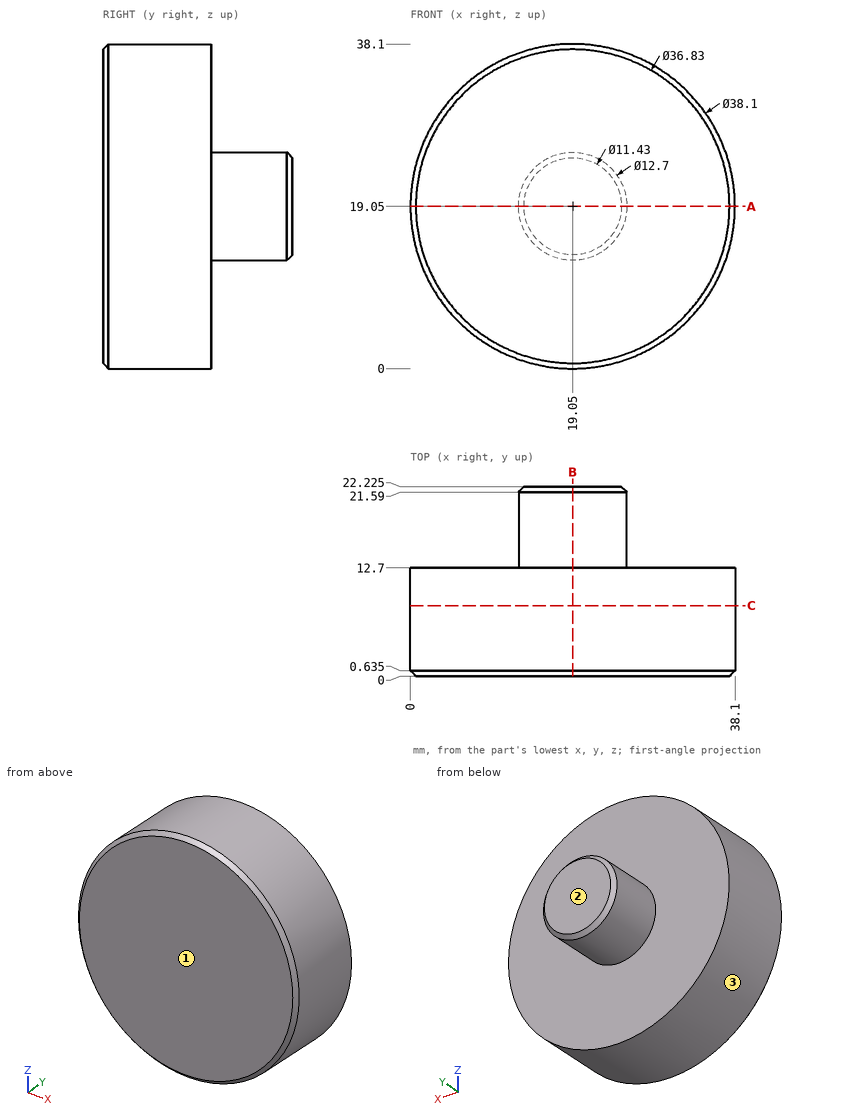
Check sheet for the drawn part. Datum: minimum x, y, z corner. Units: mm. Coordinates: 2 decimals unless noted, no trailing zeros. Order: outer loops, then holes, each group sorted by start corner. A loop starts at its lowest first (then second) coordinate and runs counter-clockwise, first axis right, second up. Notation, with made-up numbers: M 32,13.5 L 55,13.5 A30 ccw 55,41.5 Z; hole C 1,75.25 d4. An arc over 180 degrees is marked long. One line per question, with ' | ' between items. Start each with the question number.
Item 1: Gauge pin test, flat ends, axial feed: pin 1 (5 mm diameter, centred on y = 3, z = 25.5, fed in from -X); pin 2 (8 mm diameter, centred on y = 16.5, z = 16, fed in from +X); pin 3 (3 mm diameter, centred on x = 31, z = 24, fed in from +Y). Record the tip position at first contact, or that the pin passes through.
Item 2: Cross-section at B-B on x = 19.05. Enter the section's corners in (y, z) (3 decimals), then the cut area to 3 significant figures.
Item 3: Cross-section at C-C on y = 8.25. Enter the section's corners in (x, z), then the cut area to 3 significant figures.
Item 4: Cross-section at A-A on z = 19.05. Enter the section's corners in (x, y) (3 decimals), then the cut area to 3 significant figures.
Item 5: Material ranges on L1, parallel to Y at x = 21, z = 29; L2, parallel to Y at x = 9, z = 3.5; L3, parallel to Z at x = 33.5, y = 4.5, recorded low to high. Write a range as [from, to].
Item 6: Draft check along Y on the marked faces 1, 2 and 3. Enter one of: pulls with the +Y half, pulls with the -Y half, needs draft (parallel to the pull), parting line crosses it, or undercut.
Findings:
1) pin 1: stops at x = 0.41 | pin 2: stops at x = 38.01 | pin 3: stops at y = 12.7
2) outline: M 0,0.635 L 0.635,0 L 12.7,0 L 12.7,12.7 L 21.59,12.7 L 22.225,13.335 L 22.225,24.765 L 21.59,25.4 L 12.7,25.4 L 12.7,38.1 L 0.635,38.1 L 0,37.465 Z | area: 604 mm²
3) outline: C 19.05,19.05 d38.1 | area: 1,140 mm²
4) outline: M 0,0.635 L 0.635,0 L 37.465,0 L 38.1,0.635 L 38.1,12.7 L 25.4,12.7 L 25.4,21.59 L 24.765,22.225 L 13.335,22.225 L 12.7,21.59 L 12.7,12.7 L 0,12.7 Z | area: 604 mm²
5) L1: y = [0, 12.7] | L2: y = [0.1, 12.7] | L3: z = [6.64, 31.46]
6) face 1: pulls with the -Y half | face 2: pulls with the +Y half | face 3: needs draft
